Input: part model. Units: mm. Frame: model coordinates. A direction names the side the tool comes from. Give positions to 0.01 mm unless a question says otherwise; leave off trailing zeros. Loops run counter-clockwise (first coordinate to the right, second up) from the corner with the lowest first, then second, coordinate; pieces in that order, holes last. Notation, with made-up numbers: M 4,-34 L 25,-34 A22 cw 25,5 Z; hole C 29.25,30 d2. An arc over 180 degrees is marked long. Use CSV: the item, a comma, the result in double quotes. Start each with the question number.
from build123d import *

# Parameters (mm, degrees)
F0_W     = 57
F0_H     = 27
F0_R     = 4
F5_DEPTH = 2
F4_R     = 1.5
F4_R_2   = 4
F6_DEPTH = 2
F3_R     = 1.5
F3_R_2   = 4
F7_DEPTH = 2
F8_R     = 2


with BuildPart() as f5:
    # F0 (on Top) → F5 (new body)
    with BuildSketch(Plane.XY):
        Rectangle(F0_W, F0_H)
        with BuildLine():
            ThreePointArc((-18, -10), (-20, -8), (-18, -6))
            Line((-18, -6), (18, -6))
            ThreePointArc((18, -6), (20, -8), (18, -10))
            Line((18, -10), (-18, -10))
        make_face(mode=Mode.SUBTRACT)
        with BuildLine():
            ThreePointArc((-18, -2), (-20, 0), (-18, 2))
            Line((-18, 2), (-8, 2))
            ThreePointArc((-8, 2), (-6, 0), (-8, -2))
            Line((-8, -2), (-18, -2))
        make_face(mode=Mode.SUBTRACT)
        Circle(F0_R, mode=Mode.SUBTRACT)
        with BuildLine():
            ThreePointArc((8, -2), (6, 0), (8, 2))
            Line((8, 2), (18, 2))
            ThreePointArc((18, 2), (20, 0), (18, -2))
            Line((18, -2), (8, -2))
        make_face(mode=Mode.SUBTRACT)
        with BuildLine():
            ThreePointArc((-18, 6), (-20, 8), (-18, 10))
            Line((-18, 10), (18, 10))
            ThreePointArc((18, 10), (20, 8), (18, 6))
            Line((18, 6), (-18, 6))
        make_face(mode=Mode.SUBTRACT)
    extrude(amount=F5_DEPTH)

    # F4 (on line) → F6 (join)
    with BuildSketch(Plane(origin=(-28.5, 0, 0), x_dir=(0, -1, 0), z_dir=(-1, 0, 0))):
        with BuildLine():
            Line((-13.5, 0), (13.5, 0))
            Line((13.5, 0), (13.5, 47.5))
            Line((13.5, 47.5), (7.5, 47.5))
            Line((7.5, 47.5), (3.7080992435, 47.5))
            ThreePointArc((3.7080992435, 47.5), (0, 45), (-3.7080992435, 47.5))
            Line((-3.7080992435, 47.5), (-7.5000000039, 47.5))
            Line((-7.5000000039, 47.5), (-13.5, 47.5))
            Line((-13.5, 47.5), (-13.5, 0))
        make_face()
        with Locations((0, 7.5)):
            Circle(F4_R, mode=Mode.SUBTRACT)
        with Locations((0, 15)):
            Circle(F4_R_2, mode=Mode.SUBTRACT)
        with Locations((0, 22.5)):
            Circle(F4_R, mode=Mode.SUBTRACT)
        with Locations((0, 41.5)):
            Circle(F4_R, mode=Mode.SUBTRACT)
        with BuildLine():
            Line((7.5, 47.5), (13.5, 47.5))
            ThreePointArc((13.5, 47.5), (0, 61), (-13.5, 47.5))
            Line((-13.5, 47.5), (-7.5000000039, 47.5))
            Line((-7.5000000039, 47.5), (-3.7080992435, 47.5))
            ThreePointArc((-3.7080992435, 47.5), (-0.7640690498, 52.92634671), (4, 49))
            ThreePointArc((4, 49), (3.92634671, 48.2359309502), (3.7080992435, 47.5))
            Line((3.7080992435, 47.5), (7.5, 47.5))
        make_face()
        with BuildLine():
            ThreePointArc((-6, 49), (-6.4393398296, 47.9393398268), (-7.5000000039, 47.5))
            ThreePointArc((-7.5000000039, 47.5), (-8.5606601704, 50.0606601732), (-6, 49))
        make_face(mode=Mode.SUBTRACT)
        with Locations((0, 56.5)):
            Circle(F4_R, mode=Mode.SUBTRACT)
        with BuildLine():
            ThreePointArc((9, 49), (8.5606601718, 47.9393398282), (7.5, 47.5))
            ThreePointArc((7.5, 47.5), (6.4393398282, 50.0606601718), (9, 49))
        make_face(mode=Mode.SUBTRACT)
    extrude(amount=-F6_DEPTH)

    # F3 (on line) → F7 (join)
    with BuildSketch(Plane(origin=(28.5, 0, 0), x_dir=(0, -1, 0), z_dir=(-1, 0, 0))):
        with BuildLine():
            Line((-13.5, 0), (13.5, 0))
            Line((13.5, 0), (13.5, 47.5))
            Line((13.5, 47.5), (7.5, 47.5))
            Line((7.5, 47.5), (3.7080992435, 47.5))
            ThreePointArc((3.7080992435, 47.5), (0, 45), (-3.7080992435, 47.5))
            Line((-3.7080992435, 47.5), (-7.5000000039, 47.5))
            Line((-7.5000000039, 47.5), (-13.5, 47.5))
            Line((-13.5, 47.5), (-13.5, 0))
        make_face()
        with Locations((0, 7.5)):
            Circle(F3_R, mode=Mode.SUBTRACT)
        with Locations((0, 15)):
            Circle(F3_R_2, mode=Mode.SUBTRACT)
        with Locations((0, 22.5)):
            Circle(F3_R, mode=Mode.SUBTRACT)
        with Locations((0, 41.5)):
            Circle(F3_R, mode=Mode.SUBTRACT)
        with BuildLine():
            Line((7.5, 47.5), (13.5, 47.5))
            ThreePointArc((13.5, 47.5), (0, 61), (-13.5, 47.5))
            Line((-13.5, 47.5), (-7.5000000039, 47.5))
            Line((-7.5000000039, 47.5), (-3.7080992435, 47.5))
            ThreePointArc((-3.7080992435, 47.5), (-0.7640690498, 52.92634671), (4, 49))
            ThreePointArc((4, 49), (3.92634671, 48.2359309502), (3.7080992435, 47.5))
            Line((3.7080992435, 47.5), (7.5, 47.5))
        make_face()
        with BuildLine():
            ThreePointArc((-6, 49), (-6.4393398296, 47.9393398268), (-7.5000000039, 47.5))
            ThreePointArc((-7.5000000039, 47.5), (-8.5606601704, 50.0606601732), (-6, 49))
        make_face(mode=Mode.SUBTRACT)
        with Locations((0, 56.5)):
            Circle(F3_R, mode=Mode.SUBTRACT)
        with BuildLine():
            ThreePointArc((9, 49), (8.5606601718, 47.9393398282), (7.5, 47.5))
            ThreePointArc((7.5, 47.5), (6.4393398282, 50.0606601718), (9, 49))
        make_face(mode=Mode.SUBTRACT)
    extrude(amount=F7_DEPTH)

    # F8
    f8_edges = [f5.edges().sort_by_distance(p)[0] for p in [
        (-28.5, 0, 0),
        (28.5, 0, 0),
    ]]
    fillet(f8_edges, radius=F8_R)


solid = f5.part
Item 1: Section C-C (z = 25). Output: boundary loops of the cut face in (x, y).
Item 2: First-contact query: pin 1 Ø1.5 at (x, y) = (-20.5, -1.5) entering from +Z; pin 2 Ø3.5 at (y, z) = (7.5, 49) entering from +X; pin 3 Ø5 at (x, y) = (0, 0) entering from +Z. Flat tips, straight axial feed; report the tip coordinate or a pass-through.
Item 3: Set-up query: faces 1 (the cylindrical face through (-6, 0, 1)), 2 (the flat face through (-0.4, -5.8, 2)), 3 (the cylindrical face through (-28, 0, 61)). Return all of +Z, -Z, +X, -X, +Y, -Y with unobstructed straight access to the full face (end or side cutting, diameter ignored); none if empty.
Item 4: Mould query, pull axis Z, two halves, no side actions, for faces 4 (the cylindrical face through (-20, 8, 1)), 5 (the cylindrical face through (28, 0, 58)), 6 (the cylindrical face through (28, 0, 61)). Classes: +Z half, -Z half, draft (parallel to the pull), parting line (faces both ways), or undercut.
Item 5: Material intervals for line 1 (X direction, y = 6, z = 45); line 2 (Z direction, x = 25.5, y = -10.25); line 3 (Y direction, x = 27, z = 7), sorted ascending.
Item 6: Section A-A (z = 41.5). Output: boundary loops of the cut face in (x, y).
Item 7: Section B-B (x = 0). Output: boundary loops of the cut face in (y, z).
Item 8: Section D-D (x = 23.5). Output: boundary loops of the cut face in (y, z), then the cut area to 3 significant figures.
Recorded:
1,outline,"M -28.5,-13.5 L -26.5,-13.5 L -26.5,13.5 L -28.5,13.5 Z; M 26.5,-13.5 L 28.5,-13.5 L 28.5,13.5 L 26.5,13.5 Z"
2,pin 1,"z = 2"
2,pin 2,"x = 28.5"
2,pin 3,"through"
3,face 1,"+Z, -Z"
3,face 2,"+Z, +Y, -Y"
3,face 3,"+Z, +X, -X"
4,face 4,"draft"
4,face 5,"undercut"
4,face 6,"+Z half"
5,line 1,"-28.5 to -26.5, 26.5 to 28.5"
5,line 2,"0 to 2"
5,line 3,"-13.5 to -1.41, 1.41 to 13.5"
6,outline,"M -28.5,-13.5 L -26.5,-13.5 L -26.5,-1.5 L -28.5,-1.5 Z; M -28.5,1.5 L -26.5,1.5 L -26.5,13.5 L -28.5,13.5 Z; M 26.5,-13.5 L 28.5,-13.5 L 28.5,-1.5 L 26.5,-1.5 Z; M 26.5,1.5 L 28.5,1.5 L 28.5,13.5 L 26.5,13.5 Z"
7,outline,"M -13.5,0 L -10,0 L -10,2 L -13.5,2 Z; M -6,0 L -4,0 L -4,2 L -6,2 Z; M 4,0 L 6,0 L 6,2 L 4,2 Z; M 10,0 L 13.5,0 L 13.5,2 L 10,2 Z"
8,outline,"M -13.5,0 L 13.5,0 L 13.5,2 L -13.5,2 Z"
8,area,"54.0 mm²"
